```python
from build123d import *

# Parameters (mm, degrees)
SKETCH1_R           = 6
SKETCH1_R_2         = 5
BOSS_EXTRUDE1_DEPTH = 10


with BuildPart() as part:
    # Sketch1 → Boss-Extrude1 (new body)
    with BuildSketch(Plane.XY):
        with BuildLine():
            Line((10, 70), (50, 70))
            Line((50, 70), (94.685564793, 51.047419724))
            ThreePointArc((94.685564793, 51.047419724), (102, 40), (94.685564793, 28.952580276))
            Line((94.685564793, 28.952580276), (50, 10))
            Line((50, 10), (10, 10))
            Line((10, 10), (10, 30))
            Line((10, 30), (30, 30))
            ThreePointArc((30, 30), (40, 40), (30, 50))
            Line((30, 50), (10, 50))
            Line((10, 50), (10, 70))
        make_face()
        with Locations((90, 40)):
            Circle(SKETCH1_R, mode=Mode.SUBTRACT)
        with Locations((20, 60)):
            Circle(SKETCH1_R_2, mode=Mode.SUBTRACT)
        with Locations((40, 60)):
            Circle(SKETCH1_R_2, mode=Mode.SUBTRACT)
        with Locations(Location((40, 20, 0), (0, 0, 180))):
            Circle(SKETCH1_R_2, mode=Mode.SUBTRACT)
        with Locations(Location((20, 20, 0), (0, 0, 180))):
            Circle(SKETCH1_R_2, mode=Mode.SUBTRACT)
    extrude(amount=BOSS_EXTRUDE1_DEPTH)


solid = part.part
```
The model under review builds one solid part; all positions refer to its coordinate system, in mm. A direction names the side the tool comes from. Coordinates: 2 decimals unless noted, no trailing zeros. Write each loop counter-clockwise with the first axis right and the second up, starting at its lowest first coordinate (ties: lowest second). Pieces come first, ordered by that corner, then holes.
1) We need section D-D on x = 90. State the section outline as (y, z) points.
2) We need section A-A on y = 40. State the section outline as (x, z) points, then the cut area to 3 significant figures.
3) Machinability: for faces 1 (the face through (20, 30, 5)), 2 (the face through (21.08, 24.88, 4.93)), which of the approach directions +Z, -Z, +X, -X, +Y, -Y give a long, thin tool a straight path to every point of the face, cutting with its end or side? Answer none if there is none.
4) To check wall thickness, follow probe 1 along Y at (x, z) = (20, 3); probe 2 along Y at (x, z) = (18, 0.5); probe 3 along X at (y, z) = (20, 3.75). State the ranges of each line that lie inside material, in increasing order.
5) Clearance check with flat-ended pins moving along their axes: pin 1 Ø3 at (y, z) = (33, 3.5) entering from +X; pin 2 Ø1 at (x, y) = (91.5, 46) entering from -Z; pin 3 Ø1.5 at (y, z) = (31.5, 5.5) entering from -X; pin 4 Ø3 at (x, z) = (89.5, 2) entering from -Y. State where each tip first meets the part, or that it passes through.
6) The part is to be moulded in two halves that separate along Y. For faces 3 (the face through (72.66, 19.61, 4.93)), 4 (the face through (72.03, 60.656, 4.93)), 5 (the face through (23, 64, 5)), 6 (the face through (57, 40, 0)), say which applies: pulls with the +Y half, pulls with the -Y half, needs draft (parallel to the pull), parting line crosses it, or undercut.
7) We need section B-B on z = 6.5. State the section outline as (x, y) points.
8) We need section C-C on x = 20. State the section outline as (y, z) points, then the cut area to 3 significant figures.
Answer list:
1. outline: (26.97, 0) - (34, 0) - (34, 10) - (26.97, 10) - close; (46, 0) - (53.03, 0) - (53.03, 10) - (46, 10) - close
2. outline: (40, 0) - (84, 0) - (84, 10) - (40, 10) - close; (96, 0) - (102, 0) - (102, 10) - (96, 10) - close
2. area: 500 mm2
3. face 1: +Z, -Z, -X
3. face 2: +Z, -Z
4. probe 1: y = 10 to 15, 25 to 30, 50 to 55, 65 to 70
4. probe 2: y = 10 to 15.42, 24.58 to 30, 50 to 55.42, 64.58 to 70
4. probe 3: x = 10 to 15, 25 to 35, 45 to 73.58
5. pin 1: stops at x = 100.67
5. pin 2: stops at z = 0
5. pin 3: stops at x = 33.8
5. pin 4: stops at y = 26.12
6. face 3: pulls with the -Y half
6. face 4: pulls with the +Y half
6. face 5: undercut
6. face 6: needs draft
7. outline: (10, 10) - (50, 10) - (94.69, 28.95) arc R12 ccw to (94.69, 51.05) - (50, 70) - (10, 70) - (10, 50) - (30, 50) arc R10 cw to (30, 30) - (10, 30) - close; hole circle Ø10 at (20, 20); hole circle Ø10 at (20, 60); hole circle Ø10 at (40, 20); hole circle Ø10 at (40, 60); hole circle Ø12 at (90, 40)
8. outline: (10, 0) - (15, 0) - (15, 10) - (10, 10) - close; (25, 0) - (30, 0) - (30, 10) - (25, 10) - close; (50, 0) - (55, 0) - (55, 10) - (50, 10) - close; (65, 0) - (70, 0) - (70, 10) - (65, 10) - close
8. area: 200 mm2
